Here's how the part is built. I have some questions about the finished solid (model axes, mm). A direction names the side the tool comes from. Coordinates: 2 decimals unless noted, no trailing zeros. Write each loop counter-clockwise with the first axis right and the second up, starting at its lowest first coordinate (ties: lowest second). Pieces come first, ordered by that corner, then holes. Notation, with made-up numbers: (17.5, 81) - (23.5, 81) arc R10 cw to (23.5, 89) - close; hole circle Ø7 at (-30, -33). An arc over 180 degrees is marked (long way). Answer in a Markdown table with one row per item. Add a question column.
Item 1: I'm going to push flat-ended pins straight in: pin 1 (1.2 mm diameter, centred on x = 37.5, z = 3, fed in from +Y); pin 2 (1.6 mm diameter, centred on x = 20.5, z = 3.5, fed in from -Y); pin 3 (1 mm diameter, centred on y = -7.5, z = 2, fed in from -X). Where does each tip first touch, or does it pass through?
Item 2: Imagine slicing it at C-C (y = -22). Please give me the cut outline in (x, z).
Item 3: If I drill on probe 1 along X at (y, z) = (0.5, 5.15); probe 2 along Y at (x, z) = (-9.5, 2.3); probe 3 along X at (y, z) = (-10.5, 4.9), over which ranges is the centre line in solid material (lowest first)? Write a range as from..to.
Item 4: Imagine slicing it at B-B (x = 15.5). Please give me the cut outline in (y, z), plus the area to 3 significant figures.
Item 5: Which directions (+Z, -Z, +X, -X, +Y, -Y) give clear straight access to the entire face, cutting with the end or side of a thin tool? Please do faces 4 (the face through (33, 6, 3)), 5 (the face through (20, -7.4, 3)), 6 (the face through (20.9, -3, 3)).
Item 6: Imagine slicing it at A-A (y = -40). Please give me the cut outline in (x, z).
Item 7: Imagine slicing it at D-D (z = 5.15). State how many separate pieces and enclosed holes the cut face has, plus the area to 3 significant figures.
Item 8: We'd pull the mould along X, two halves only. Please class faces 1 (the face through (1, -13, 0)), 2 (the face through (26, -5, 3)), 3 (the face through (-11.91, -44.38, 2.96)): +X half, -X half, draft (parallel to the pull), parting line (faces both ways), or undercut.
from build123d import *

# Parameters (mm, degrees)
SKETCH_1_R           = 2.05
EXTRUDE_1_DEPTH      = 6
SKETCH_2_W           = 7
SKETCH_2_H           = 6
EXTRUDE_2_DEPTH      = 6
CUT_EXTRUDE_1_DEPTH  = 7
SKETCH_21_W          = 7
SKETCH_21_H          = 6
EXTRUDE_21_DEPTH     = 6
SKETCH_22_W          = 7
SKETCH_22_H          = 6
EXTRUDE_22_DEPTH     = 6
CUT_EXTRUDE_12_DEPTH = 7


with BuildPart() as part:
    # Эскиз1 → Бобышка-Вытянуть1 (new body)
    with BuildSketch(Plane.XY):
        with BuildLine():
            Line((-40, 0), (40, 0))
            Line((40, 0), (13.757679871, -42.621480902))
            ThreePointArc((13.757679871, -42.621480902), (11.938503177, -44.365054668), (9.5, -45))
            Line((9.5, -45), (-9.5, -45))
            ThreePointArc((-9.5, -45), (-11.938503177, -44.365054668), (-13.757679871, -42.621480902))
            Line((-13.757679871, -42.621480902), (-40, 0))
        make_face()
        with Locations((-9.5, -40)):
            Circle(SKETCH_1_R, mode=Mode.SUBTRACT)
        with Locations((9.5, -40)):
            Circle(SKETCH_1_R, mode=Mode.SUBTRACT)
        with BuildLine():
            Line((-17.17379907, -15), (17.17379907, -15))
            ThreePointArc((17.17379907, -15), (19.792831871, -16.536898094), (19.728406993, -19.572888541))
            Line((19.728406993, -19.572888541), (10.829793891, -34.025576661))
            ThreePointArc((10.829793891, -34.025576661), (9.738287875, -35.071720921), (8.275185968, -35.45268812))
            Line((8.275185968, -35.45268812), (-8.275185968, -35.45268812))
            ThreePointArc((-8.275185968, -35.45268812), (-9.738287875, -35.071720921), (-10.829793891, -34.025576661))
            Line((-10.829793891, -34.025576661), (-19.728406993, -19.572888541))
            ThreePointArc((-19.728406993, -19.572888541), (-19.792831871, -16.536898094), (-17.17379907, -15))
        make_face(mode=Mode.SUBTRACT)
    extrude(amount=EXTRUDE_1_DEPTH)

    # Эскиз2 → Бобышка-Вытянуть2 (add)
    with BuildSketch(Plane(origin=(-23, -50, 0), x_dir=(-1, 0, 0), z_dir=(0, 0, -1))):
        with Locations((-9.531849908, 53)):
            Rectangle(SKETCH_2_W, SKETCH_2_H)
        with Locations((9.531849908, 53)):
            Rectangle(SKETCH_2_W, SKETCH_2_H)
    extrude(amount=-EXTRUDE_2_DEPTH)

    # Эскиз3 → Вырез-Вытянуть1 (cut, through all)
    with BuildSketch(Plane(origin=(-23, -50, 0), x_dir=(-1, 0, 0), z_dir=(0, 0, -1))):
        Polygon((-2.1, 45), (-3.6, 45), (-3.6, 42.6), (-2.1, 42.6), (-2.1, 39), (2.1, 39), (2.1, 42.6), (3.6, 42.6), (3.6, 45), (2.1, 45), (2.1, 50), (-2.1, 50), align=None)
    extrude(amount=-CUT_EXTRUDE_1_DEPTH, mode=Mode.SUBTRACT)

    # Эскиз21 → Бобышка-Вытянуть21 (add)
    with BuildSketch(Plane(origin=(-23, -50, 6), x_dir=(1, 0, 0), z_dir=(0, 0, 1))):
        with Locations((-9.531849908, 53)):
            Rectangle(SKETCH_21_W, SKETCH_21_H)
        with Locations((9.531849908, 53)):
            Rectangle(SKETCH_21_W, SKETCH_21_H)
    extrude(amount=-EXTRUDE_21_DEPTH)

    # Эскиз22 → Бобышка-Вытянуть22 (add)
    with BuildSketch(Plane(origin=(23, -50, 0), x_dir=(-1, 0, 0), z_dir=(0, 0, -1))):
        with Locations((-9.531849908, 53)):
            Rectangle(SKETCH_22_W, SKETCH_22_H)
        with Locations((9.531849908, 53)):
            Rectangle(SKETCH_22_W, SKETCH_22_H)
    extrude(amount=-EXTRUDE_22_DEPTH)

    # Эскиз32 → Вырез-Вытянуть12 (cut, through all)
    with BuildSketch(Plane(origin=(23, -50, 0), x_dir=(-1, 0, 0), z_dir=(0, 0, -1))):
        Polygon((-2.1, 45), (-3.6, 45), (-3.6, 42.6), (-2.1, 42.6), (-2.1, 39), (2.1, 39), (2.1, 42.6), (3.6, 42.6), (3.6, 45), (2.1, 45), (2.1, 50), (-2.1, 50), align=None)
    extrude(amount=-CUT_EXTRUDE_12_DEPTH, mode=Mode.SUBTRACT)


solid = part.part
Here are the results:
| question | item | result |
|---|---|---|
| 1 | pin 1 | stops at y = 0 |
| 1 | pin 2 | stops at y = -32.97 |
| 1 | pin 3 | stops at x = -35.69 |
| 2 | outline | (-26.45, 0) - (-18.23, 0) - (-18.23, 6) - (-26.45, 6) - close; (18.23, 0) - (26.45, 0) - (26.45, 6) - (18.23, 6) - close |
| 3 | probe 1 | x = -36.03..-29.03, -16.97..-9.97, 9.97..16.97, 29.03..36.03 |
| 3 | probe 2 | y = -45..-42.05, -37.95..-35.19, -15..0 |
| 3 | probe 3 | x = -33.54..-25.1, -20.9..20.9, 25.1..33.54 |
| 4 | outline | (-39.79, 0) - (-26.44, 0) - (-26.44, 6) - (-39.79, 6) - close; (-15, 0) - (6, 0) - (6, 6) - (-15, 6) - close |
| 4 | area | 206 mm2 |
| 5 | face 4 | +Z, -Z, +X, -X, +Y |
| 5 | face 5 | +Z, -Z |
| 5 | face 6 | +Z, -Z, +Y |
| 6 | outline | (-15.37, 0) - (-11.55, 0) - (-11.55, 6) - (-15.37, 6) - close; (-7.45, 0) - (7.45, 0) - (7.45, 6) - (-7.45, 6) - close; (11.55, 0) - (15.37, 0) - (15.37, 6) - (11.55, 6) - close |
| 7 | separate pieces | 1 |
| 7 | enclosed holes | 3 |
| 7 | area | 1,730 mm2 |
| 8 | face 1 | draft |
| 8 | face 2 | undercut |
| 8 | face 3 | -X half |
